Check sheet for the drawn part. Datum: minimum x, y, z corner. Units: mm. A direction names the side the tool comes from. Give positions to 0.01 mm unless a question says otherwise; leave off trailing zeros. Loops run counter-clockwise (first coordinate to the right, second up) from the corner with the lowest first, then second, coordinate; pieces in that order, holes last. Notation, with made-up numbers: (-8, -22) - (20, -22) arc R28 cw to (20, 14) - close; hole circle Ø10 at (37.25, 53). An arc over 180 degrees is marked (long way). One line per item, written item: value. Start each with the question number.
1. Scan lines: L1, parallel to X at y = 18, z = 36.5; L2, parallel to Y at x = 19, z = 8; L3, parallel to X at y = 30, z = 13. Record each from-to range of solid material in increasing order. Write a range as [from, to].
2. Sectioned sample at D-D (x = 21.5). Record the cut outline in (y, z), plus the area to 3 significant figures.
3. Gauge pin test, flat ends, axial feed: pin 1 (10 mm diameter, centred on y = 26.5, z = 5, fed in from -X); pin 2 (10 mm diameter, centred on x = 20.5, z = 27, fed in from +Y). Record the tip position at first contact, or that the pin passes through.
4. Sectioned sample at B-B (x = 52.5). Record the cut outline in (y, z), plus the area to 3 significant figures.
5. Access from +Z, -Z, +X, -X, +Y, -Y to the whole of each face (thin tool, end or side, straight path). Record for the marked faces 1, 2, 3 and 4.
6. Sectioned sample at C-C (y = 8.5). Record the cut outline in (x, z).
7. Sectioned sample at A-A (z = 37.5). Record the cut outline in (x, y), plus the area to 3 significant figures.
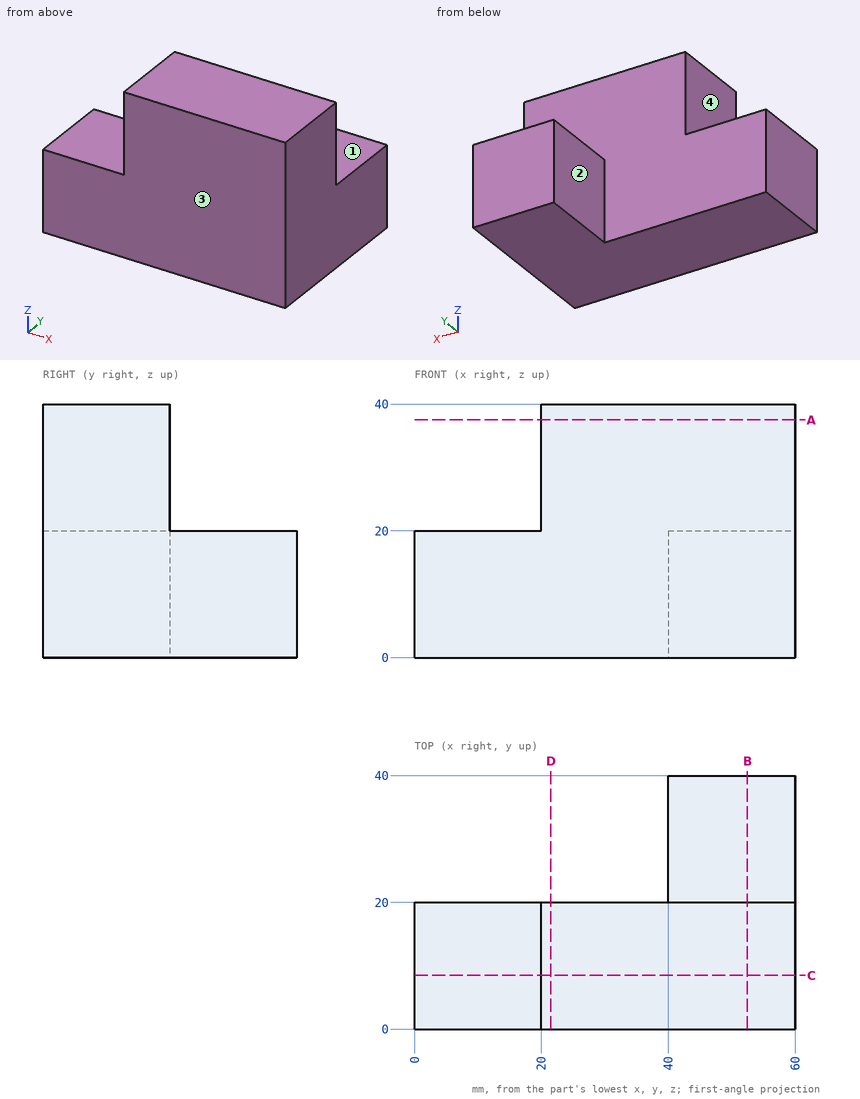
Results are:
1. L1: x = [20, 60]
1. L2: y = [0, 20]
1. L3: x = [40, 60]
2. outline: (0, 0) - (20, 0) - (20, 40) - (0, 40) - close
2. area: 800 mm^2
3. pin 1: stops at x = 40
3. pin 2: stops at y = 20
4. outline: (0, 0) - (40, 0) - (40, 20) - (20, 20) - (20, 40) - (0, 40) - close
4. area: 1,200 mm^2
5. face 1: +Z, +X, -X, +Y
5. face 2: +Z, -Z, -X, +Y
5. face 3: +Z, -Z, +X, -X, -Y
5. face 4: +Z, -X, +Y, -Y
6. outline: (0, 0) - (60, 0) - (60, 40) - (20, 40) - (20, 20) - (0, 20) - close
7. outline: (20, 0) - (60, 0) - (60, 20) - (20, 20) - close
7. area: 800 mm^2
